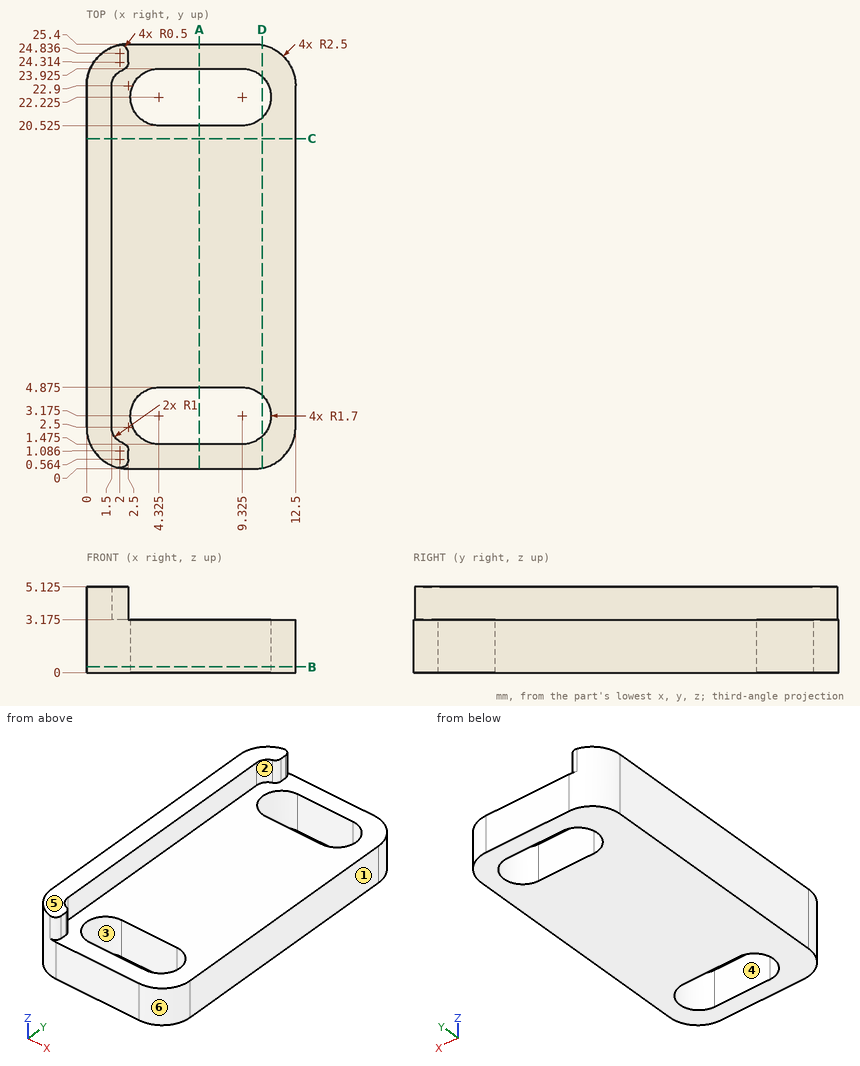
Design review of the part shown in the three views and the two pictorial views. Dimensions are in mm from the part's minimum x, y and z. A direction names the side the tool comes from. Round coordinates to 2 decimals unless told otherwise and drop trailing zeros. Order: outer loops, then holes, each group sorted by start corner. A loop starts at its lowest first (then second) coordinate and runs counter-clockwise, first axis right, second up. Notation, with made-up numbers: M 44.25,-38.5 L 61.25,-38.5 A24 ccw 61.25,-15.5 Z; hole C 85,-34.75 d4. An arc over 180 degrees is marked long. Put each result on its own line as item: value.
Q1. Consider section C-C (y = 19.75). State the section outline as (x, z) points (1 decimal).
Reported:
outline: M 0,0 L 12.5,0 L 12.5,3.2 L 1.5,3.2 L 1.5,5.1 L 0,5.1 Z
Q2. Consider section D-D (x = 10.5). State how many separate pieces and enclosed holes the cut face has.
Reported:
separate pieces: 3
enclosed holes: 0
Q3. Consider section B-B (z = 0.35). State the section outline as (x, y) points (1 decimal).
Reported:
outline: M 0,2.5 A2.5 ccw 2.5,0 L 10,0 A2.5 ccw 12.5,2.5 L 12.5,22.9 A2.5 ccw 10,25.4 L 2.5,25.4 A2.5 ccw 0,22.9 Z; hole M 4.3,1.5 L 9.3,1.5 A1.7 ccw 9.3,4.9 L 4.3,4.9 A1.7 ccw Z; hole M 4.3,20.5 L 9.3,20.5 A1.7 ccw 9.3,23.9 L 4.3,23.9 A1.7 ccw Z
Q4. Draft analysis for pull direction Y (two halves, no side actions). For the marked faces 4, 5 and 6, state which applies: released by +Y, released by -Y, zero draft, split by the parting line, or undercut.
Reported:
face 4: undercut
face 5: zero draft
face 6: released by -Y
Q5. Insertion check: pin 1 Ø3.5 at (x, y) = (8, 16.5) entering from +Z (1 decimal); pin 2 Ø0.6 at (y, z) = (24.5, 4) entering from +X; pin 3 Ø0.6 at (y, z) = (12, 4.5) entering from +X. Each pin has a flat end and moves straight along its axis. Give the tip position at first contact, or say it passes through.
Reported:
pin 1: z = 3.2
pin 2: x = 2.5
pin 3: x = 1.5
Q6. To check wall thickness, follow line 1 (Y direction, x = 6.5, z = 1.05) (1 decimal); line 2 (Z direction, x = 12, y = 14) (1 decimal); line 3 (X direction, y = 16, z = 4.7). State the ranges of each line that lie inside material, in increasing order.
Reported:
line 1: 0 to 1.5, 4.9 to 20.5, 23.9 to 25.4
line 2: 0 to 3.2
line 3: 0 to 1.5
Q7. Machinability: for the marked faces 1, 2 and 3, which of the approach directions +Z, -Z, +X, -X, +Y, -Y give a long, thin tool a straight path to every point of the face, cutting with its end or side? Answer none if there is none.
Reported:
face 1: +Z, -Z, +X, +Y, -Y
face 2: +Z, +X
face 3: +Z, -Z
Q8. Consider section A-A (x = 6.75). State the section outline as (y, z) points (1 decimal).
Reported:
outline: M 0,0 L 1.5,0 L 1.5,3.2 L 0,3.2 Z; M 4.9,0 L 20.5,0 L 20.5,3.2 L 4.9,3.2 Z; M 23.9,0 L 25.4,0 L 25.4,3.2 L 23.9,3.2 Z
